The drawing under review shows one solid part. Ordinate dimensions are in mm from its lowest x, y, z. A direction names the side the tool comes from. Give positions to 0.01 mm unless a question says otherwise; leave off trailing zeros. Loops run counter-clockwise (first coordinate to the right, second up) from the corner with the lowest first, then second, coordinate; pieces in that order, holes last. Notation, with made-up numbers: (80, 58) -> (115, 58) arc R20 ccw to (115, 64) -> close; hole circle Ø5 at (38.5, -32). An arc over 180 degrees is marked (long way). Answer in a Markdown table with one row per item. Add a question column.
(1) Consider section A-A on x = 2.25. Write out the cut boundary in (y, z), then the cut area to 3 significant figures.
(2) Draft analysis for pull direction Y (two halves, no side actions). For the marked faces 1, 2, 3 and 4, state which applies: +Y half, -Y half, draft (parallel to the pull), parting line (faces both ways), or undercut.
(3) Consider section C-C on y = 0.75. Write out the cut boundary in (x, z).
(4) For line 1 (X direction, y = 1.8, z = 2.25); line 2 (Y direction, x = 3.15, z = 4.15); line 3 (Z direction, x = 2.25, y = 3.4), list the stretches that pass through material, from the lowest coordinate up.
(5) For the marked faces 5 and 6, list the 3-axis set-ups (+Z, -Z, +X, -X, +Y, -Y) from which the entire face can be reached by the end or side of a thin tool; tool diameter is ignored.
(6) Consider section D-D on x = 3.9. Write out the cut boundary in (y, z), then the cut area to 3 significant figures.
(7) Consider section B-B on z = 2.25. Write out the cut boundary in (x, y).
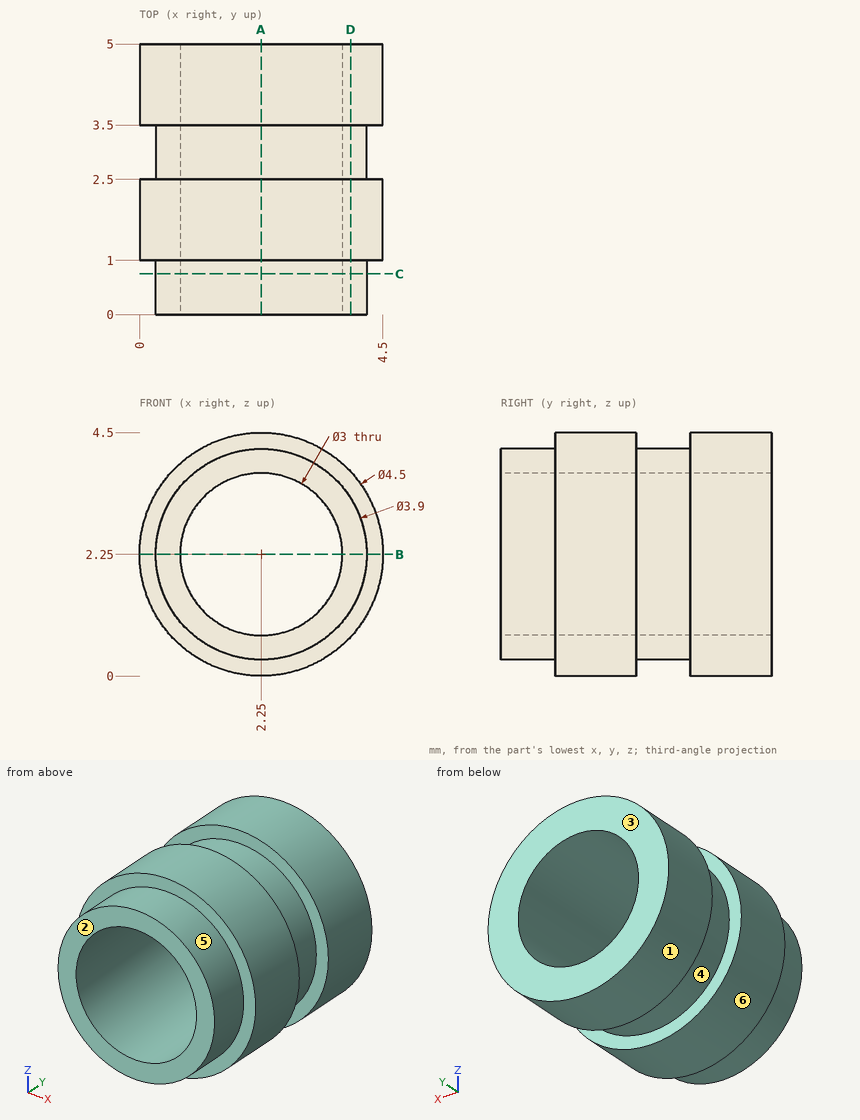
Values follow:
| question | item | result |
|---|---|---|
| 1 | outline | (0, 0.3) -> (1, 0.3) -> (1, 0) -> (2.5, 0) -> (2.5, 0.3) -> (3.5, 0.3) -> (3.5, 0) -> (5, 0) -> (5, 0.75) -> (0, 0.75) -> close; (0, 3.75) -> (5, 3.75) -> (5, 4.5) -> (3.5, 4.5) -> (3.5, 4.2) -> (2.5, 4.2) -> (2.5, 4.5) -> (1, 4.5) -> (1, 4.2) -> (0, 4.2) -> close |
| 1 | area | 6.30 mm2 |
| 2 | face 1 | draft |
| 2 | face 2 | -Y half |
| 2 | face 3 | +Y half |
| 2 | face 4 | undercut |
| 3 | outline | circle Ø3.9 at (2.25, 2.25); hole circle Ø3 at (2.25, 2.25) |
| 4 | line 1 | 0 to 0.75, 3.75 to 4.5 |
| 4 | line 2 | 1 to 2.5, 3.5 to 5 |
| 4 | line 3 | 0.3 to 0.75, 3.75 to 4.2 |
| 5 | face 5 | -Y |
| 5 | face 6 | +Y, -Y |
| 6 | outline | (0, 1.21) -> (1, 1.21) -> (1, 0.72) -> (2.5, 0.72) -> (2.5, 1.21) -> (3.5, 1.21) -> (3.5, 0.72) -> (5, 0.72) -> (5, 3.78) -> (3.5, 3.78) -> (3.5, 3.29) -> (2.5, 3.29) -> (2.5, 3.78) -> (1, 3.78) -> (1, 3.29) -> (0, 3.29) -> close |
| 6 | area | 13.3 mm2 |
| 7 | outline | (0, 1) -> (0.3, 1) -> (0.3, 0) -> (0.75, 0) -> (0.75, 5) -> (0, 5) -> (0, 3.5) -> (0.3, 3.5) -> (0.3, 2.5) -> (0, 2.5) -> close; (3.75, 0) -> (4.2, 0) -> (4.2, 1) -> (4.5, 1) -> (4.5, 2.5) -> (4.2, 2.5) -> (4.2, 3.5) -> (4.5, 3.5) -> (4.5, 5) -> (3.75, 5) -> close |
